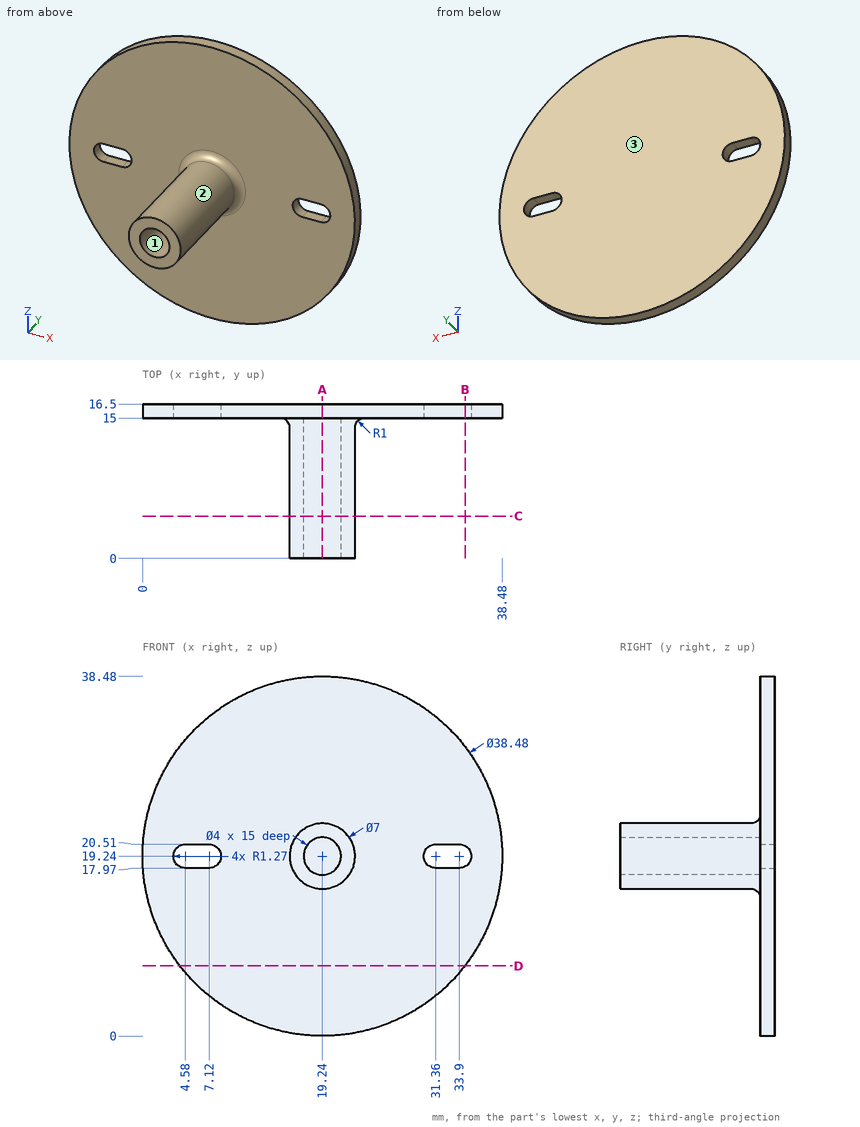
The drawing under review shows one solid part. Ordinate dimensions are in mm from its lowest x, y, z. Give positions to 0.01 mm unless a question says otherwise; leave off trailing zeros. Write each loop counter-clockwise with the first axis right and the second up, starting at its lowest first coordinate (ties: lowest second). Pieces come first, ordered by that corner, then holes. Notation, with made-up numbers: (26.5, 80.5) -> (45.5, 80.5) arc R22 ccw to (45.5, 87.5) -> close; hole circle Ø9 at (-27, -2.5). An arc over 180 degrees is marked (long way). Use CSV: the item, a comma, the result in double quotes.
Q1. For P1, Ø1.6, axis at x = 6, y = 15.5, coming from the +Z side; P2, Ø4, axis at x = 9, z = 4, coming from the -Y side; P3, Ø8, axis at y = 11.5, z = 17.5, coming from the +X side, all flat-tipped, find the tip position at first contact; note any pin that passes through.
Conclusion:
P1,"z = 33.92"
P2,"y = 15"
P3,"x = 38.48"
Q2. Take a section at A-A, the plane x = 19.24. Write out the cut boundary in (y, z), then the cut area to 3 significant figures.
Conclusion:
outline,"(0, 15.74) -> (14, 15.74) arc R1 cw to (15, 14.74) -> (15, 0) -> (16.5, 0) -> (16.5, 38.48) -> (15, 38.48) -> (15, 23.74) arc R1 cw to (14, 22.74) -> (0, 22.74) -> (0, 21.24) -> (15, 21.24) -> (15, 17.24) -> (0, 17.24) -> close"
area,"103 mm2"
Q3. Mouldability with a two-part tool opening along Z and no side actions: class the marked faces 1, 2 and 3 as pulls with the +Z half, pulls with the -Z half, needs draft (parallel to the pull), parting line crosses it, or undercut.
Conclusion:
face 1,"undercut"
face 2,"parting line crosses it"
face 3,"needs draft"
Q4. Take a section at C-C, the plane y = 4.5. Write out the cut boundary in (x, z), then the cut area to 3 significant figures.
Conclusion:
outline,"circle Ø7 at (19.24, 19.24); hole circle Ø4 at (19.24, 19.24)"
area,"25.9 mm2"
Q5. To check wall thickness, follow probe 1 along X at (y, z) = (10, 19.24); probe 2 along Y at (x, z) = (24.5, 16); probe 3 along X at (y, z) = (10.5, 19). State the ranges of each line that lie inside material, in increasing order. Write a range as [from, to].
Conclusion:
probe 1,"[15.74, 17.24], [21.24, 22.74]"
probe 2,"[15, 16.5]"
probe 3,"[15.75, 17.25], [21.23, 22.73]"
Q6. Take a section at B-B, the plane x = 34.5. Write out the cut boundary in (y, z), then the cut area to 3 significant figures.
Conclusion:
outline,"(15, 7.52) -> (16.5, 7.52) -> (16.5, 18.12) -> (15, 18.12) -> close; (15, 20.36) -> (16.5, 20.36) -> (16.5, 30.96) -> (15, 30.96) -> close"
area,"31.8 mm2"
Q7. Take a section at D-D, the plane z = 7.5. Write out the cut boundary in (x, y).
Conclusion:
outline,"(4, 15) -> (34.48, 15) -> (34.48, 16.5) -> (4, 16.5) -> close"
